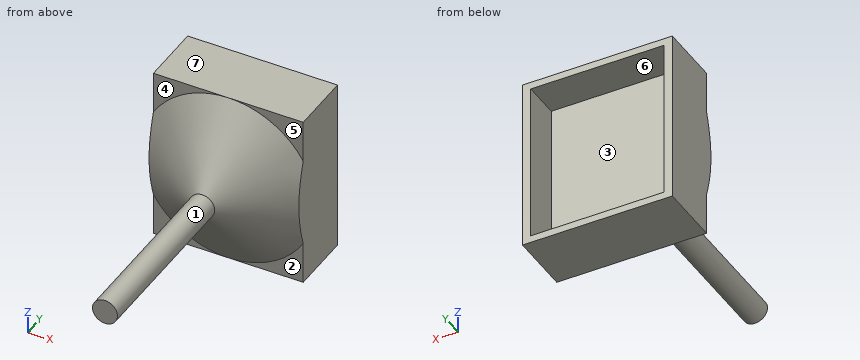
from build123d import *

# Parameters (mm, degrees)
SKETCH1_R               = 5
BOSS_EXTRUDE1_DEPTH     = 90
BOSS_EXTRUDE2_START     = 90
SKETCH2_W               = 60
SKETCH2_H               = 70
BOSS_EXTRUDE2_DEPTH     = 25
CUT_EXTRUDE1_DEPTH      = 126.199840255
CUT_EXTRUDE1_DEPTH_BACK = 126.199840255
SKETCH5_W               = 76.98796528
SKETCH5_H               = 79.307753312
SKETCH5_W_2             = 60
SKETCH5_H_2             = 70
CUT_EXTRUDE2_START      = 115
SKETCH6_W               = 53.399999872
SKETCH6_H               = 64.250000016
CUT_EXTRUDE2_DEPTH      = 15


with BuildPart() as part:
    # Sketch1 → Boss-Extrude1 (new body)
    with BuildSketch(Plane(origin=(0, 0, 0), x_dir=(1, 0, 0), z_dir=(0, 1, 0))):
        with Locations(Location((0, 0, 0), (0, 0, 90))):
            Circle(SKETCH1_R)
    extrude(amount=BOSS_EXTRUDE1_DEPTH)

    # Sketch2 → Boss-Extrude2 (add)
    with BuildSketch(Plane(origin=(0, 0, 0), x_dir=(1, 0, 0), z_dir=(0, 1, 0)).offset(BOSS_EXTRUDE2_START)):
        Rectangle(SKETCH2_W, SKETCH2_H)
    extrude(amount=BOSS_EXTRUDE2_DEPTH)

    # Sketch4 → Revolve1 (revolve)
    with BuildSketch(Plane(origin=(0, 0, 0), x_dir=(0, 0, -1), z_dir=(1, 0, 0)), mode=Mode.PRIVATE) as revolve1_sk:
        Polygon((-35, 90), (-5, 70.95), (-5, 90), align=None)
    revolve(revolve1_sk.sketch.rotate(Axis((0, 90, 0), (0, -1, 0)), 180), axis=Axis((0, 90, 0), (0, -1, 0)))

    # Sketch5 → Cut-Extrude1 (cut, two sides: drawn at the far end of the back side and taken through both)
    with BuildSketch(Plane(origin=(0, 0, 0), x_dir=(1, 0, 0), z_dir=(0, 1, 0)).offset(-CUT_EXTRUDE1_DEPTH_BACK)):
        Rectangle(SKETCH5_W, SKETCH5_H)
        Rectangle(SKETCH5_W_2, SKETCH5_H_2, mode=Mode.SUBTRACT)
    extrude(amount=CUT_EXTRUDE1_DEPTH + CUT_EXTRUDE1_DEPTH_BACK, mode=Mode.SUBTRACT)

    # Sketch6 → Cut-Extrude2 (cut)
    with BuildSketch(Plane(origin=(0, 0, 0), x_dir=(1, 0, 0), z_dir=(0, 1, 0)).offset(CUT_EXTRUDE2_START)):
        Rectangle(SKETCH6_W, SKETCH6_H)
    extrude(amount=-CUT_EXTRUDE2_DEPTH, mode=Mode.SUBTRACT)


solid = part.part
Input: part model. Units: mm. Frame: model coordinates. Face numbers are marked on the shaded views. A direction names the side the tool comes from. Coordinates: 2 decimals unless noted, no trailing zeros. Order: outer loops, then holes, each group sorted by start corner. A loop starts at its lowest first (then second) coordinate and runs counter-clockwise, first axis right, second up. Notation, with made-up numbers: M 51,67 L 94,67 A19 cw 94,81 Z; hole C -4.5,-32.75 d10. An arc over 180 degrees is marked long. Write item = value, one per line. Start each with the question number.
(1) Pull-direction query (Z, two-part tool) for the marked faces 5, 6 and 7; classes: released by +Z, released by -Z, zero draft, split by the parting line, or undercut.
(2) First-contact query: P1, Ø6, axis at x = 1.5, y = 19, coming from the -Z side; P2, Ø8.5, axis at x = 14.5, z = 24.5, coming from the -Y side; P3, Ø5, axis at x = -9.5, z = 30.5, coming from the -Y side. Flat tips, straight axial feed; report the tip coordinate or a pass-through.
(3) Section C-C on y = 82.5. Output: boundary loops of the cut face in (x, z), and give its area (3 significant figures).
(4) Line query: line 1 along Z through (x, y) = (-3, 106) (3 decimals); line 2 along Y through (x, z) = (-23.5, 30); line 3 along X through (y, z) = (27, 0.5). Output: solid intervals per line, ascending. Write a range as [from, to].
(5) Reachability of the marked faces 1, 2, 3 and 4 from +Z, -Z, +X, -X, +Y, -Y: full face, straight path, thin tool, end or side. Return the list, or none.
(6) Section B-B on y = 13.5. Output: boundary loops of the cut face in (x, z).
(7) Section A-A on z = 0. Output: boundary loops of the cut face in (x, y) (3 decimals).
Result set:
q1.face_5 = zero draft
q1.face_6 = undercut
q1.face_7 = released by +Z
q2.P1 = -5
q2.P2 = 83.15
q2.P3 = 86.47
q3.outline = C 0,0 d46.38
q3.area = 1,690 mm²
q4.line_1 = [-35, -32.125], [32.125, 35]
q4.line_2 = [90, 100]
q4.line_3 = [-4.97, 4.97]
q5.face_1 = -Y
q5.face_2 = -Z, +X, -Y
q5.face_3 = +Y
q5.face_4 = +Z, -X, -Y
q6.outline = C 0,0 d10
q7.outline = M -30,86.825 L -5,70.95 L -5,0 L 5,0 L 5,70.95 L 30,86.825 L 30,115 L 26.7,115 L 26.7,100 L -26.7,100 L -26.7,115 L -30,115 Z
